The model under review builds one solid part; all positions refer to its coordinate system, in mm. A direction names the side the tool comes from. Coordinates: 2 decimals unless noted, no trailing zeros. Write each loop counter-clockwise with the first axis right and the second up, starting at its lowest first coordinate (ties: lowest second). Pieces come first, ordered by that corner, then holes.
1) Add section A-A, the plane x = 37.5. State the section outline as (y, z) points.
2) Add section B-B, the plane x = 93. State the section outline as (y, z) points, then the cut area to 3 significant figures.
3) Mouldability with a two-part tool opening along Z and no side actions: class faces 5 (the flat face through (74, 11, -117)), 6 (the flat face through (112, 40, -3)), 7 (the flat face through (40, 8, -120)), 8 (the cylindrical face through (20.01, 1.48, -103.61)) as released by +Z, released by -Z, zero draft, split by the parting line, or undercut.
4) For P1, Ø3.5, axis at x = 141, z = -102.5, coming from the +Y side; P2, Ø3, axis at x = 36, y = 11.5, coming from the +Z side; P3, Ø11, axis at x = 112, y = 31, coming from the -Z side, all flat-tipped, find the tip position at first contact; note any pin that passes through.
5) Machinability: for faces 1 (the flat face through (115, 8, -120)), 2 (the flat face through (110, 28, -3)), 3 (the flat face through (74, 20, -120)), 4 (the flat face through (75, 21, -3)), which of the approach directions +Z, -Z, +X, -X, +Y, -Y give a long, thin tool a straight path to every point of the face, cutting with its end or side? Answer none if there is none.
6) For line 1 (Z direction, x = 141, y = 1.2); line 2 (X direction, y = 1.7, z = -20.5); line 3 (Y direction, x = 112.5, z = -119.1), list the stretches that pass through material, from the lowest coordinate up.
7) Add section C-C, the plane z = -92.5. State the section outline as (x, y) points, then the cut area to 3 significant figures.
from build123d import *

# Parameters (mm, degrees)
SKETCH_1_W          = 150
SKETCH_1_H          = 123
SKETCH_1_R          = 1.5
EXTRUDE_1_DEPTH     = 3
SKETCH_2_W          = 150
SKETCH_2_H          = 6
EXTRUDE_2_DEPTH     = 17
SKETCH_3_W          = 75
SKETCH_3_H          = 6
EXTRUDE_3_DEPTH     = 37
CUT_EXTRUDE_1_DEPTH = 37
SKETCH_5_R          = 5
CUT_EXTRUDE_2_DEPTH = 3
CUT_EXTRUDE_3_DEPTH = 6
SKETCH_7_R          = 5
CUT_EXTRUDE_4_DEPTH = 3


with BuildPart() as part:
    # 草图1 → 凸台-拉伸1 (new body)
    with BuildSketch(Plane(origin=(0, 0, 0), x_dir=(1, 0, 0), z_dir=(0, 1, 0))):
        with Locations((75, 61.5)):
            Rectangle(SKETCH_1_W, SKETCH_1_H)
        with Locations(Location((19, 102.5, 0), (0, 0, 270))):
            Circle(SKETCH_1_R, mode=Mode.SUBTRACT)
        with Locations(Location((19, 20.5, 0), (0, 0, 270))):
            Circle(SKETCH_1_R, mode=Mode.SUBTRACT)
        with Locations(Location((141, 20.5, 0), (0, 0, 270))):
            Circle(SKETCH_1_R, mode=Mode.SUBTRACT)
        with Locations(Location((141, 102.5, 0), (0, 0, 270))):
            Circle(SKETCH_1_R, mode=Mode.SUBTRACT)
    extrude(amount=EXTRUDE_1_DEPTH)

    # 草图2 → 凸台-拉伸2 (add)
    with BuildSketch(Plane(origin=(0, 3, 0), x_dir=(1, 0, 0), z_dir=(0, 1, 0))):
        with Locations((75, 120)):
            Rectangle(SKETCH_2_W, SKETCH_2_H)
    extrude(amount=EXTRUDE_2_DEPTH)

    # 草图3 → 凸台-拉伸3 (add)
    with BuildSketch(Plane(origin=(0, 3, 0), x_dir=(1, 0, 0), z_dir=(0, 1, 0))):
        with Locations((112.5, 3)):
            Rectangle(SKETCH_3_W, SKETCH_3_H)
    extrude(amount=EXTRUDE_3_DEPTH)

    # 草图4 → 切除-拉伸1 (cut)
    with BuildSketch(Plane(origin=(0, 0, -6), x_dir=(-1, 0, 0), z_dir=(0, 0, -1))):
        with BuildLine():
            ThreePointArc((-109.987789157, 30.669922891), (-113.169922891, 32.512210843), (-115.012210843, 29.330077109))
            Line((-115.012210843, 29.330077109), (-109.987789157, 30.669922891))
        make_face()
        with BuildLine():
            Line((-109.987789157, 30.669922891), (-115.012210843, 29.330077109))
            ThreePointArc((-115.012210843, 29.330077109), (-112.162174743, 27.422040711), (-109.9, 30))
            ThreePointArc((-109.9, 30), (-109.922040711, 30.337825257), (-109.987789157, 30.669922891))
        make_face()
    extrude(amount=-CUT_EXTRUDE_1_DEPTH, mode=Mode.SUBTRACT)

    # 草图5 → 切除-拉伸2 (cut)
    with BuildSketch(Plane(origin=(0, 0, -6), x_dir=(-1, 0, 0), z_dir=(0, 0, -1))):
        with Locations((-112.5, 30)):
            Circle(SKETCH_5_R)
    extrude(amount=-CUT_EXTRUDE_2_DEPTH, mode=Mode.SUBTRACT)

    # 草图6 → 切除-拉伸3 (cut)
    with BuildSketch(Plane(origin=(0, 0, -123), x_dir=(-1, 0, 0), z_dir=(0, 0, -1))):
        with BuildLine():
            ThreePointArc((-115.1, 10), (-112.5, 7.4), (-109.9, 10))
            Line((-109.9, 10), (-115.1, 10))
        make_face()
        with BuildLine():
            Line((-115.1, 10), (-109.9, 10))
            ThreePointArc((-109.9, 10), (-112.5, 12.6), (-115.1, 10))
        make_face()
        with BuildLine():
            ThreePointArc((-34.9, 10), (-37.5, 12.6), (-40.1, 10))
            Line((-40.1, 10), (-34.9, 10))
        make_face()
        with BuildLine():
            Line((-34.9, 10), (-40.1, 10))
            ThreePointArc((-40.1, 10), (-37.5, 7.4), (-34.9, 10))
        make_face()
    extrude(amount=-CUT_EXTRUDE_3_DEPTH, mode=Mode.SUBTRACT)

    # 草图7 → 切除-拉伸4 (cut)
    with BuildSketch(Plane.XY.offset(-117)):
        with Locations((37.5, 10)):
            Circle(SKETCH_7_R)
        with Locations((112.5, 10)):
            Circle(SKETCH_7_R)
    extrude(amount=-CUT_EXTRUDE_4_DEPTH, mode=Mode.SUBTRACT)


solid = part.part
Geometry results:
1. outline: (0, -123) - (7.4, -123) - (7.4, -120) - (5, -120) - (5, -117) - (3, -117) - (3, 0) - (0, 0) - close; (12.6, -123) - (20, -123) - (20, -117) - (15, -117) - (15, -120) - (12.6, -120) - close
2. outline: (0, -123) - (20, -123) - (20, -117) - (3, -117) - (3, -6) - (40, -6) - (40, 0) - (0, 0) - close
2. area: 693 mm2
3. face 5: undercut
3. face 6: zero draft
3. face 7: released by +Z
3. face 8: undercut
4. P1: stops at y = 3
4. P2: stops at z = -120
4. P3: stops at z = -6
5. face 1: none
5. face 2: -Z
5. face 3: -Z, +X, -X, +Y
5. face 4: +Z, -X, +Y
6. line 1: z = -123 to -104, -101 to -22, -19 to 0
6. line 2: x = 0 to 17.5, 20.5 to 139.5, 142.5 to 150
6. line 3: y = 0 to 5, 15 to 20
7. outline: (0, 0) - (150, 0) - (150, 3) - (0, 3) - close
7. area: 450 mm2
